```python
from build123d import *

# Parameters (mm, degrees)
BOSS_EXTRUDE1_DEPTH = 2
BOSS_EXTRUDE2_DEPTH = 10
CUT_EXTRUDE1_REACH  = 522
BOSS_EXTRUDE3_DEPTH = 2


with BuildPart() as part:
    # Sketch1 → Boss-Extrude1 (new body)
    with BuildSketch(Plane(origin=(0, 0, 0), x_dir=(1, 0, 0), z_dir=(0, 1, 0))):
        Polygon((-49.497474683, -516.187950266), (233.345237792, -233.345237792), (0, 0), (-282.842712475, -282.842712475), align=None)
    extrude(amount=BOSS_EXTRUDE1_DEPTH)

    # Sketch4 → Boss-Extrude2 (add)
    with BuildSketch(Plane(origin=(0, 2, 0), x_dir=(1, 0, 0), z_dir=(0, 1, 0))):
        Polygon((3.535533906, -10.606601718), (-3.535533906, -17.67766953), (215.667568262, -236.880771697), (222.738636074, -229.809703886), align=None)
    extrude(amount=BOSS_EXTRUDE2_DEPTH)

    # Sketch6 → Cut-Extrude1 (cut, up to next)
    with BuildSketch(Plane(origin=(7.071067812, 0, 7.071067812), x_dir=(-0.707106781, 0, 0.707106781), z_dir=(-0.707106781, 0, -0.707106781)), mode=Mode.PRIVATE) as cut_extrude1_sk1:
        with BuildLine():
            Line((5, 12), (5, 7))
            ThreePointArc((5, 7), (6.464466094, 10.535533906), (10, 12))
            Line((10, 12), (5, 12))
        make_face()
    cut_extrude1_tool1 = extrude(cut_extrude1_sk1.sketch, amount=-CUT_EXTRUDE1_REACH, mode=Mode.PRIVATE) & part.part
    add(cut_extrude1_tool1.solids().sort_by_distance((2.745809, 10.88316, 11.396327))[0], mode=Mode.SUBTRACT)
    # Sketch6 → Cut-Extrude1 (cut, up to next)
    with BuildSketch(Plane(origin=(7.071067812, 0, 7.071067812), x_dir=(-0.707106781, 0, 0.707106781), z_dir=(-0.707106781, 0, -0.707106781)), mode=Mode.PRIVATE) as cut_extrude1_sk2:
        with BuildLine():
            Line((15, 12), (10, 12))
            ThreePointArc((10, 12), (13.535533906, 10.535533906), (15, 7))
            Line((15, 7), (15, 12))
        make_face()
    cut_extrude1_tool2 = extrude(cut_extrude1_sk2.sketch, amount=-CUT_EXTRUDE1_REACH, mode=Mode.PRIVATE) & part.part
    add(cut_extrude1_tool2.solids().sort_by_distance((-2.745809, 10.88316, 16.887945))[0], mode=Mode.SUBTRACT)

    # Sketch10 → Boss-Extrude3 (add)
    with BuildSketch(Plane(origin=(0, 0, 0), x_dir=(1, 0, 0), z_dir=(0, 1, 0))):
        Polygon((-282.842712475, -282.842712475), (-516.187950266, -516.187950266), (-49.497474683, -516.187950266), align=None)
    extrude(amount=BOSS_EXTRUDE3_DEPTH)


solid = part.part
```
Geometry check sheet. Reference: the model listing, model coordinates, mm. A direction names the side the tool comes from. Round coordinates to 2 decimals unless told otherwise and drop trailing zeros. Loops run counter-clockwise (first coordinate to the right, second up) from the corner with the lowest first, then second, coordinate; pieces in that order, holes last. Notation, with made-up numbers: (70.5, 74.25) - (98.5, 74.25) arc R36 cw to (98.5, 108.25) - close; hole circle Ø7 at (-7, -24). An arc over 180 degrees is marked (long way). Write item = value, one per line. Start each with the question number.
1. Section check A-A on x = -145.5. Enter the section's corners in (y, z).
2. Thickness scan on line 1 (Y direction, x = 20, z = 251.5); line 2 (Z direction, x = -448, y = 1.25); line 3 (X direction, y = 10.25, z = 138). Record the ranges inside material, lowest first.
3. Set-up check for faces 1 (the face through (89.94, 0.99, 376.75)), 2 (the face through (114.67, 4.46, 121.74)), 3 (the face through (104.532, 4.465, 125.745)): record each of +Z, -Z, +X, -X, +Y, -Y from which the full face is reachable in a straight line by a thin tool's end or side.
4. Section check B-B on z = 348. Enter the section's corners in (x, y), then the cut area to 3 significant figures.
5. Depth check by flat-ended pin: pin 1 (5 mm diameter, centred on x = 86, z = 158, fed in from +Y); pin 2 (2 mm diameter, centred on y = 1.5, z = 462.5, fed in from -X); pin 3 (4 mm diameter, centred on y = 6.5, z = 146.5, fed in from -X). Enter the tip coordinate at first touch or a pass-through.
Working result:
q1.outline = (0, 145.5) - (2, 145.5) - (2, 516.19) - (0, 516.19) - close
q2.line_1 = 0 to 2
q2.line_2 = 448 to 516.19
q2.line_3 = 118.48 to 129.23
q3.face_1 = +Z, +X, +Y, -Y
q3.face_2 = -Z, +X, +Y
q3.face_3 = +Z, -X, +Y
q4.outline = (-348, 0) - (118.69, 0) - (118.69, 2) - (-348, 2) - close
q4.area = 933 mm^2
q5.pin_1 = 2
q5.pin_2 = -463.5
q5.pin_3 = 123.29
